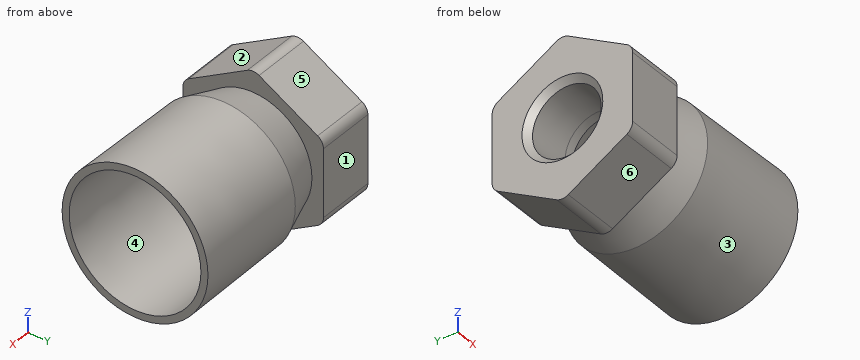
Autodesk Inventor part; units mm, degrees
ref_plane "YZ Plane" through (0, 0, 0) normal (1, 0, 0) x (0, 1, 0)
ref_plane "XZ Plane" through (0, 0, 0) normal (0, 1, 0) x (-1, 0, 0)
ref_plane "XY Plane" through (0, 0, 0) normal (0, 0, 1) x (1, 0, 0)
sketch "Sketch1" plane through (0, 0, 0) normal (0, 0, 1) x (1, 0, 0)
  line L0 (0, 0) -> (6.6144, 0) construction
  line L1 (0, 0) -> (0, 4.75) construction
  line L2 (0, 4.75) -> (8, 4.3864)
  line L3 (6.6144, 0) -> (16.6144, 0) construction
  line L4 (16.6144, 0) -> (16.6144, 12.2) construction
  line L5 (16.6144, 0) -> (36.6144, 0) construction
  line L6 (36.6144, 0) -> (36.6144, 12.45) construction
  line L7 (36.6144, 12.45) -> (16.6144, 12.2)
  line L8 (0, 4.75) -> (0, 6.75)
  line L9 (0, 4.75) -> (2, 4.75) construction
  line L10 (0, 6.75) -> (16.6144, 12.2)
  line L11 (8, 4.3864) -> (16.6144, 11)
  line L12 (16.6144, 11) -> (36.6144, 11.2499)
  line L13 (36.6144, 11.2499) -> (36.6144, 12.45)
  line L14 (0, 0) -> (3.3, 0) construction
  line L15 (3.3, 0) -> (3.3, 4.6) construction
  dimension "d2" = 4.75
  dimension "d3" = 12.2
  dimension "d4" = 20
  dimension "d5" = 12.45
  dimension "d6" = 2
  dimension "d7" = 90
  dimension "d8" = 1.2
  dimension "d9" = 1.2
  dimension "d10" = 10
  dimension "d24" = 177.397
  dimension "d25" = 8
  dimension "d26" = 3.3
  dimension "d27" = 4.6
  dimension "d28" = 6.6144
revolve "Revolution1" add sketch "Sketch1" angle 360 about axis through (6.6144, 0, 0) along (1, 0, 0)
sketch "Sketch2" plane through (0, 0, 0) normal (-1, 0, 0) x (0, 0, 1)
  circle A0 centre (0, 0) radius 6.75
  line L0 (0, -6.75) -> (0, -12.2) construction
  circle A1 centre (0, 0) radius 12.2
  line L1 (1.633, -6.5495) -> (2.9514, -11.8376)
  line L2 (-1.633, -6.5495) -> (-2.9514, -11.8376)
  point P0 (-1.633, -6.5495)
  point P1 (-2.9514, -11.8376)
  dimension "d12" = 14
extrude "Extrusion1" [suppressed]
chamfer "Chamfer1" [suppressed]
pattern_circular "Circular Pattern1" [suppressed]
chamfer "Chamfer2" distance 0.7 angle 45 1 edges at (0, -4.75, 0)
sketch "Sketch3" plane through (0, 0, 0) normal (-1, 0, 0) x (0, 0, 1)
  line L0 (-6.9282, -12) -> (-13.8564, 0)
  line L1 (-13.8564, 0) -> (-6.9282, 12)
  line L2 (-6.9282, 12) -> (6.9282, 12)
  line L3 (6.9282, 12) -> (13.8564, 0)
  line L4 (13.8564, 0) -> (6.9282, -12)
  line L5 (6.9282, -12) -> (-6.9282, -12)
  circle A0 centre (0, 0) radius 6.75
  point P0 (0, -12)
  dimension "d32" = 24
extrude "Extrusion2" add sketch "Sketch3" against normal blind 10
fillet "Fillet1" radius 2 6 edges at (5, 12, 6.9282) (5, 12, -6.9282) (5, 0, -13.8564) (5, -12, -6.9282) (5, -12, 6.9282) (5, 0, 13.8564)
sketch "Sketch4" plane through (0, 0, 0) normal (0, 1, 0) x (-1, 0, 0)
  line L0 (-8, 4.3864) -> (-8, -4.3864)
  line L1 (0, 0) -> (-8, 0)
  line L2 (-8, 0) -> (-8, -5.6) construction
  line L3 (-8, -5.6) -> (0, -5.6) construction
  line L4 (0, -5.6) -> (0, 0)
  line L5 (-8, -5.6) -> (0, -5.6) construction
  line L6 (0, -5.6) -> (0, -5.9)
  line L7 (0, -5.9) -> (-8, -5.9) construction
  line L8 (-8, -5.9) -> (-8, -5.6)
  line L9 (-8, -5.6) -> (0, -5.9)
  line L10 (-16.6144, 11) -> (-16.6144, -11)
  line L11 (-8, 4.3864) -> (-8, -4.3864)
  line L12 (-16.6144, -11) -> (-8, -4.3864)
  line L13 (-8, -5.6) -> (-9.5072, -5.5435)
  line L14 (-8, 0) -> (-8, -4.3864)
  line L15 (-8, -4.3864) -> (-9.5072, -5.5435)
  dimension "d33" = 5.6
  dimension "d34" = 0.3
revolve "Revolution2" cut sketch "Sketch4" angle 360 about axis through (0, 0, 0) along (1, 0, 0)
chamfer "Chamfer3" distance 1 angle 45 1 edges at (0, 0, 5.9)
equation "\"Tol\" = 0"
properties part number "PneumaticAdaptorFemale"
Geometry: final body of the model. Coordinates: model frame, mm. Face numbers are marked on the shaded views. A direction names the side the tool comes from. Give positions to 0.01 mm unless a question says otherwise; leave off trailing zeros. Loops run counter-clockwise (first coordinate to the right, second up) from the corner with the lowest first, then second, coordinate; pieces in that order, holes last. Notation, with made-up numbers: M 61,56.25 L 93,56.25 A31 cw 93,87.25 Z; hole C 6.25,-32.75 d1. An arc over 180 degrees is marked long. Put each result on its own line as item: value. Start each with the question number.
1) Contact query for flat-ended pins moving along their axis: pin 1 (11 mm diameter, centred on x = 7.5, z = -1.5, fed in from -Y); pin 2 (3 mm diameter, centred on x = 16, z = -3, fed in from +Y); pin 3 (7 mm diameter, centred on y = -1, z = -2.5, fed in from +X). Output: stop coordinate, or through.
2) Access query for the marked faces 1, 2 and 3. Directions: +Z, -Z, +X, -X, +Y, -Y. A direction counts if a zero-diameter tool reaches every point of the face in a straight line with its end or side. Return the directions, or none.
3) Ray query, line 1 along Z through (x, y) = (20, -1); line 2 along X through (y, z) = (10.75, 7.25); line 3 along Z through (x, y) = (16, -7.25). Return the intervals inside material, ascending.
4) Cut plane B-B (x = 28). Output: boundary loops of the cut face in (y, z), then the cut area to 3 significant figures.
5) Cut plane A-A (x = 13). Output: boundary loops of the cut face in (y, z).
6) Pull-direction query (Y, two-part tool) for the marked faces 4, 5 and 6; classes: pulls with the +Y half, pulls with the -Y half, needs draft (parallel to the pull), parting line crosses it, or undercut.
Verdict:
1. pin 1: y = -12
1. pin 2: y = 12.09
1. pin 3: x = 10.35
2. face 1: +Z, -Z, -X, +Y
2. face 2: +Z, -X, -Y
2. face 3: none
3. line 1: -12.2 to -11, 11 to 12.2
3. line 2: 0 to 10
3. line 3: -9.56 to -7.63, 7.63 to 9.56
4. outline: C 0,0 d24.68; hole C 0,0 d22.28
4. area: 88.5 mm2
5. outline: C 0,0 d22.03; hole C 0,0 d16.45
6. face 4: undercut
6. face 5: pulls with the +Y half
6. face 6: pulls with the -Y half
